Geometry: final body of the model. Coordinates: model frame, mm. Give positions to 0.01 mm unless a question says otherwise; leave off trailing zeros. Loops run counter-clockwise (first coordinate to the right, second up) from the corner with the lowest first, then second, coordinate; pieces in that order, holes last.
Autodesk Inventor part; units mm, degrees
ref_plane "YZ Plane" through (0, 0, 0) normal (1, 0, 0) x (0, 1, 0)
ref_plane "XZ Plane" through (0, 0, 0) normal (0, 1, 0) x (-1, 0, 0)
ref_plane "XY Plane" through (0, 0, 0) normal (0, 0, 1) x (1, 0, 0)
sketch "Sketch1" plane through (0, 0, 0) normal (0, 0, 1) x (1, 0, 0)
  circle A0 centre (0, 0) radius 37.25
  circle A1 centre (0, 0) radius 12
  dimension "d0" = 74.5
  dimension "d1" = 24
extrude "Extrusion1" add sketch "Sketch1" along normal blind 10
sketch "Sketch7" plane through (0, 0, 10) normal (0, 0, 1) x (1, 0, 0)
  circle A0 centre (0, 0) radius 22
  circle A1 centre (0, 0) radius 38
  dimension "d32" = 44
  dimension "d33" = 76
extrude "Extrusion6" cut sketch "Sketch7" against normal blind 6.35 contours A0 | A1
sketch "Sketch9" plane through (0, 0, 3.65) normal (0, 0, 1) x (1, 0, 0)
  circle A0 centre (30, 0) radius 1
  circle A1 centre (24.2705, 17.6336) radius 1
  circle A2 centre (9.2705, 28.5317) radius 1
  circle A3 centre (-9.2705, 28.5317) radius 1
  circle A4 centre (-24.2705, 17.6336) radius 1
  circle A5 centre (-30, 0) radius 1
  circle A6 centre (-24.2705, -17.6336) radius 1
  circle A7 centre (-9.2705, -28.5317) radius 1
  circle A8 centre (9.2705, -28.5317) radius 1
  circle A9 centre (24.2705, -17.6336) radius 1
  point P0 (0, 0)
  dimension "d44" = 2
  dimension "d45" = 30
  dimension "d48" = 360
extrude "Extrusion8" cut sketch "Sketch9" against normal through all
sketch "Sketch10" plane through (0, 0, 3.65) normal (0, 0, 1) x (1, 0, 0)
  circle A0 centre (30, 0) radius 1
  circle A1 centre (30, 0) radius 1
  circle A2 centre (30, 0) radius 2
  circle A3 centre (24.2705, 17.6336) radius 2
  circle A4 centre (9.2705, 28.5317) radius 2
  circle A5 centre (-9.2705, 28.5317) radius 2
  circle A6 centre (-24.2705, 17.6336) radius 2
  circle A7 centre (-30, 0) radius 2
  circle A8 centre (-24.2705, -17.6336) radius 2
  circle A9 centre (-9.2705, -28.5317) radius 2
  circle A10 centre (9.2705, -28.5317) radius 2
  circle A11 centre (24.2705, -17.6336) radius 2
  point P0 (0, 0)
  dimension "d52" = 4
  dimension "d55" = 360
extrude "Extrusion9" cut sketch "Sketch10" against normal blind 2 contours A0 | A2 | A3 | A4 | A5 | A6 | A7 | A8 | A9 | A10 | A11
properties part number "SG01" material "ABS Plastic"
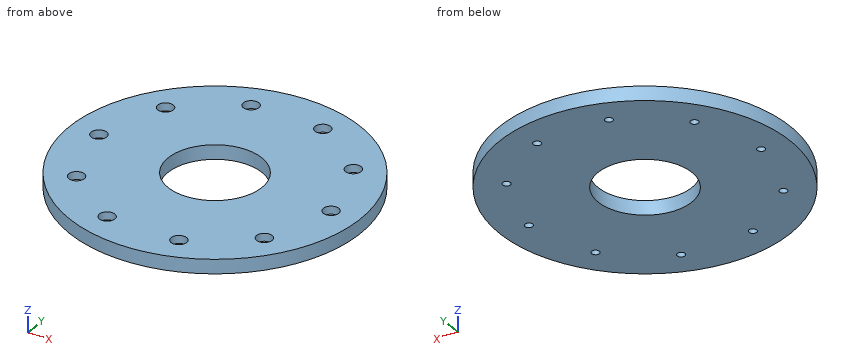
Item 1: Ray query, probe 1 along X at (y, z) = (-17, 0.3); probe 2 along Y at (x, z) = (0, 0.2); probe 3 along Y at (x, z) = (-10, 0.65). Return the intervals inside material, ascending.
Values follow:
probe 1: x = -33.14 to -25.04, -23.5 to 23.5, 25.04 to 33.14
probe 2: y = -37.25 to -12, 12 to 37.25
probe 3: y = -35.88 to -29.22, -27.85 to -6.63, 6.63 to 27.85, 29.22 to 35.88
Item 2: Section query A-A on x = 0. Return loops of the section in (y, z), plus the area to 3 significant figures.
Values follow:
outline: (-37.25, 0) - (-12, 0) - (-12, 3.65) - (-37.25, 3.65) - close; (12, 0) - (37.25, 0) - (37.25, 3.65) - (12, 3.65) - close
area: 184 mm2
Item 3: Pin query (flat end, axial travel): pin 1 (2 mm diameter, centred on x = -29.5, y = 0.5, fed in from +Z); pin 2 (2 mm diameter, centred on x = -19, z = 0.5, fed in from +Y); pin 3 (1 mm diameter, centred on y = 23, z = 1, fed in from -X). Return the tip coordinate at first contact, or that it passes through.
Values follow:
pin 1: stops at z = 1.65
pin 2: stops at y = 32.61
pin 3: stops at x = -29.69
Item 4: Section query D-D on x = -30. Return loops of the section in (y, z).
Values follow:
outline: (-22.08, 0) - (-1, 0) - (-1, 1.65) - (-2, 1.65) - (-2, 3.65) - (-22.08, 3.65) - close; (1, 0) - (22.08, 0) - (22.08, 3.65) - (2, 3.65) - (2, 1.65) - (1, 1.65) - close
Item 5: Section query C-C on z = 0.6. Give the number of separate pieces and of enclosed holes in the cut face, plus the area to 3 significant figures.
Values follow:
separate pieces: 1
enclosed holes: 11
area: 3,880 mm2
Item 6: Section query B-B on y = 0. Return loops of the section in (x, z), plus the area to 3 significant figures.
Values follow:
outline: (-37.25, 0) - (-31, 0) - (-31, 1.65) - (-32, 1.65) - (-32, 3.65) - (-37.25, 3.65) - close; (-29, 0) - (-12, 0) - (-12, 3.65) - (-28, 3.65) - (-28, 1.65) - (-29, 1.65) - close; (12, 0) - (29, 0) - (29, 1.65) - (28, 1.65) - (28, 3.65) - (12, 3.65) - close; (31, 0) - (37.25, 0) - (37.25, 3.65) - (32, 3.65) - (32, 1.65) - (31, 1.65) - close
area: 162 mm2
